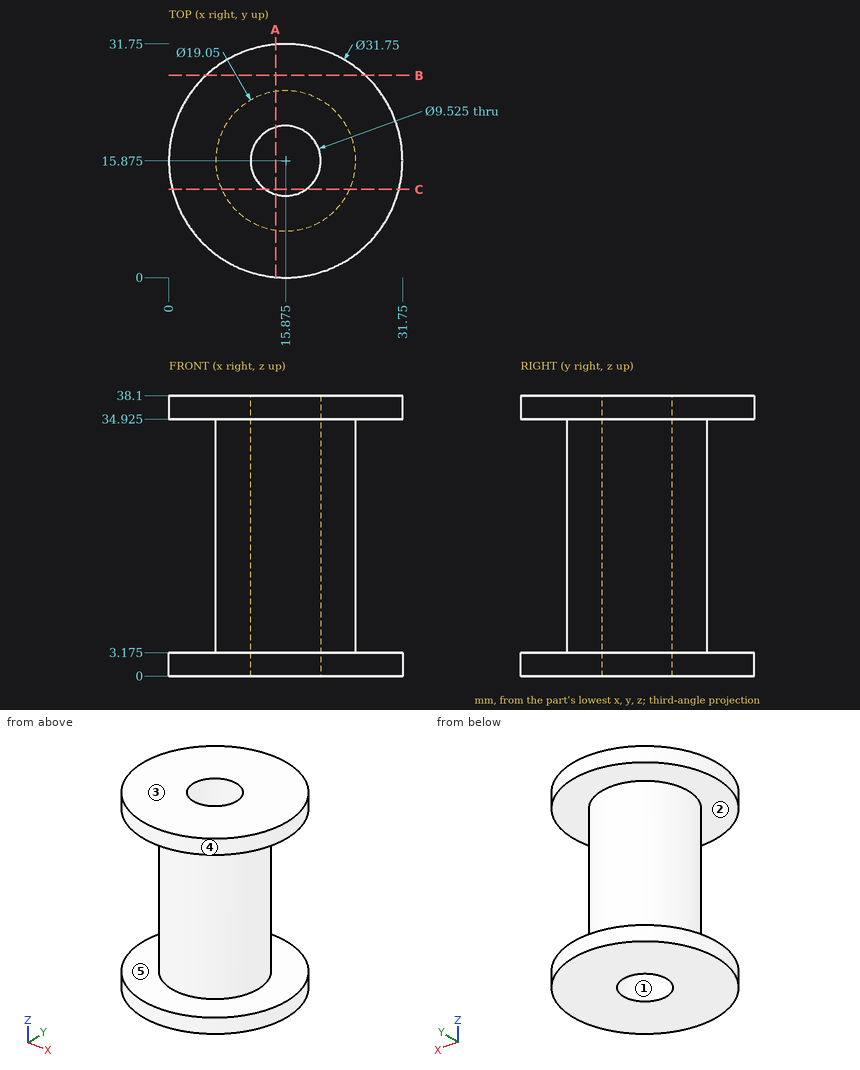
Job drawing, mm, ordinate dimensions from the low corner. One solid piece. A direction names the side the tool comes from. Give positions to 0.01 mm unless a question says otherwise; leave off trailing zeros. Write each loop counter-clockwise with the first axis right and the second up, starting at its lowest first coordinate (ties: lowest second). Pieces come first, ordered by that corner, then holes. Notation, with made-up numbers: M 68.25,15 L 119.25,15 A17 ccw 119.25,20 Z; hole C 31.5,76 d2. An arc over 180 degrees is marked long. One line per item, written item: value. Start each with the question number.
Q1. Probe probe 1 along Z at (x, y) = (5, 8) (3 decimals); probe 2 along X at (y, z) = (18.5, 27); probe 3 along Y at (x, z) = (14, 30). List the from-to ranges inside material, lowest first. Write a range as [from, to].
Q2. Drop flat-ended pins along their axis: pin 1 Ø4 at (y, z) = (18, 23.5) entering from -X; pin 2 Ø12 at (x, z) = (27.5, 26) entering from -Y; pin 3 Ø1 at (x, z) = (23, 17) entering from -Y. Give the stop position or say it passes through.
Q3. Saw through at B-B, the plane y = 27.5. Write the cut outline in (x, z) (3 decimals), plus the area to 3 significant figures.
Q4. Saw through at A-A, the plane x = 14.5. Write the cut outline in (y, z) (3 decimals).
Q5. Saw through at C-C, the plane y = 12. Write the cut outline in (x, z) (3 decimals).
Q6. Two-plate mould, pull along Z, no slides. Class the marked faces 3, 4 and 5: +Z half, -Z half, draft (parallel to the pull), parting line (faces both ways), or undercut.
Q7. 3-axis set-ups, long thin cutter, end or side, ignore diameter. For the marked faces 1 and 2: which of +Z, -Z, +X, -X, +Y, -Y reach the whole face in a straight line?
Output values:
1. probe 1: z = [0, 3.175], [34.925, 38.1]
1. probe 2: x = [6.72, 11.9], [19.85, 25.03]
1. probe 3: y = [6.54, 11.5], [20.25, 25.21]
2. pin 1: stops at x = 6.35
2. pin 2: stops at y = 8.19
2. pin 3: stops at y = 9.03
3. outline: M 5.064,0 L 26.686,0 L 26.686,3.175 L 5.064,3.175 Z; M 5.064,34.925 L 26.686,34.925 L 26.686,38.1 L 5.064,38.1 Z
3. area: 137 mm²
4. outline: M 0.06,0 L 11.315,0 L 11.315,38.1 L 0.06,38.1 L 0.06,34.925 L 6.45,34.925 L 6.45,3.175 L 0.06,3.175 Z; M 20.435,0 L 31.69,0 L 31.69,3.175 L 25.3,3.175 L 25.3,34.925 L 31.69,34.925 L 31.69,38.1 L 20.435,38.1 Z
5. outline: M 0.48,0 L 13.106,0 L 13.106,38.1 L 0.48,38.1 L 0.48,34.925 L 7.174,34.925 L 7.174,3.175 L 0.48,3.175 Z; M 18.644,0 L 31.27,0 L 31.27,3.175 L 24.576,3.175 L 24.576,34.925 L 31.27,34.925 L 31.27,38.1 L 18.644,38.1 Z
6. face 3: +Z half
6. face 4: draft
6. face 5: undercut
7. face 1: +Z, -Z
7. face 2: none
